Part print with two shaded views. Sizes in mm from the minimum x, y, z corner. A direction names the side the tool comes from. Round coordinates to 2 decimals unless told otherwise and drop trailing zeros. Write each loop counter-clockwise with the first axis right and the second up, starting at its lowest first coordinate (ties: lowest second). Pieces come first, ordered by that corner, then holes. Notation, with made-up numbers: M -6,-26.5 L 49,-26.5 A15 ccw 49,1.5 Z; hole C 49.25,-13 d7. An arc over 180 degrees is marked long. Use one line per item in the form item = value. Start each with the question number.
Item 1: Which spindle directions (+Z, -Z, +X, -X, +Y, -Y) get a long thin tool onto all of the face, cutting with end or side? Do the marked faces 1 and 2. Say none if no direction does.
Item 2: Cut at C-C, the plane z = 7.5. Give the cut face in (x, y).
Item 3: Cut at A-A, the plane y = 50.8. Give the cut face in (x, z) (3 decimals), then the cut area to 3 significant figures.
Item 4: Probe L1, parallel to Y at x = 50, z = 61; L2, parallel to Y at x = 50.8, z = 60.5 (3 decimals); L3, parallel to Z at x = 53.5, y = 33. List the from-to ranges inside material, lowest first.
Item 5: Cut at D-D, the plane z = 49.5. Give the cut face in (x, y), then the cut area to 3 significant figures.
Item 6: Flat gauge pins, fed straight in: pin 1 Ø1.9 at (x, y) = (49.5, 69.5) entering from +Z; pin 2 Ø2 at (x, y) = (75, 35.5) entering from +Z; pin 3 Ø1 at (x, z) = (23.5, 47.5) entering from +Y. Where does each tip first touch, or does it go through?
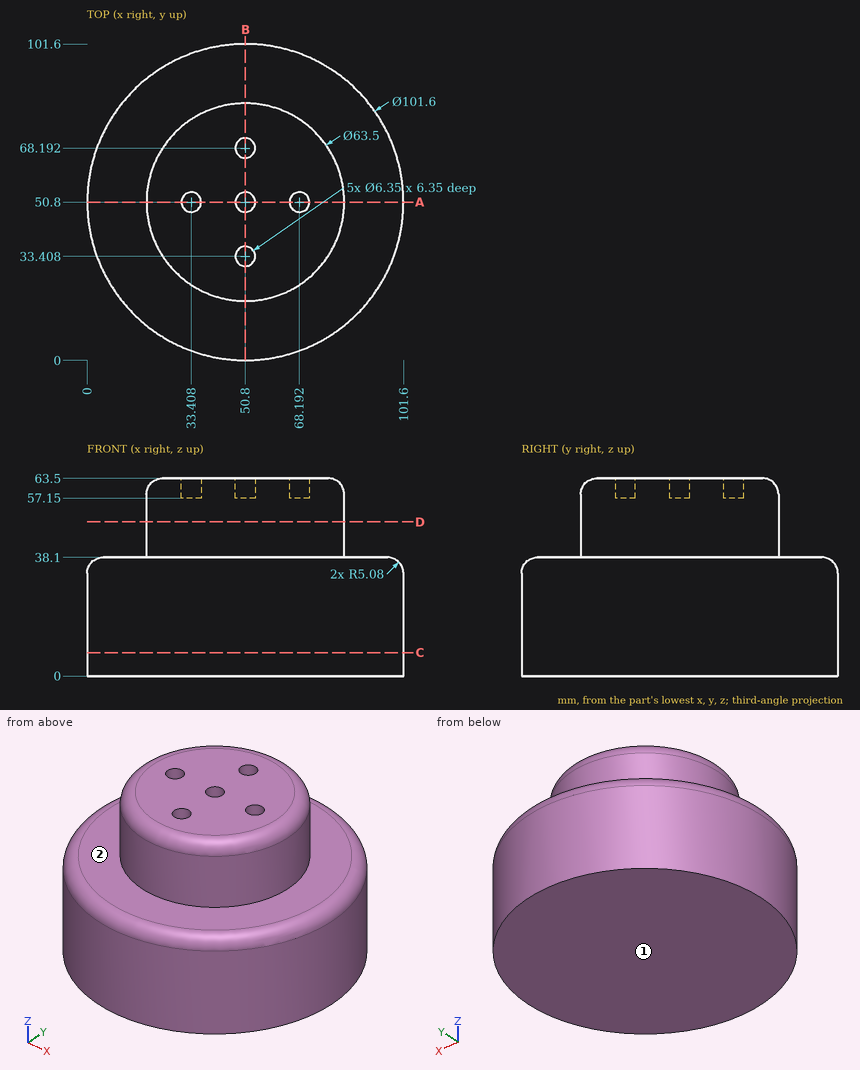
Model answer:
q1.face_1 = -Z, +X, -X, +Y, -Y
q1.face_2 = +Z
q2.outline = C 50.8,50.8 d101.6
q3.outline = M 0,0 L 101.6,0 L 101.6,33.02 A5.08 ccw 96.52,38.1 L 82.55,38.1 L 82.55,58.42 A5.08 ccw 77.47,63.5 L 71.367,63.5 L 71.367,57.15 L 65.017,57.15 L 65.017,63.5 L 53.975,63.5 L 53.975,57.15 L 47.625,57.15 L 47.625,63.5 L 36.583,63.5 L 36.583,57.15 L 30.233,57.15 L 30.233,63.5 L 24.13,63.5 A5.08 ccw 19.05,58.42 L 19.05,38.1 L 5.08,38.1 A5.08 ccw 0,33.02 Z
q3.area = 5,340 mm²
q4.L1 = 19.76 to 30.34, 36.48 to 47.73, 53.87 to 65.12, 71.26 to 81.84
q4.L2 = 19.495 to 30.233, 36.583 to 47.625, 53.975 to 65.017, 71.367 to 82.105
q4.L3 = 0 to 57.15
q5.outline = C 50.8,50.8 d63.5
q5.area = 3,170 mm²
q6.pin_1 = 57.15
q6.pin_2 = 63.41
q6.pin_3 = 67.82
